```python
from build123d import *

# Parameters (mm, degrees)
RESSALTO_EXTRUS_O1_DEPTH   = 160
ESBO_O2_W                  = 7.6
ESBO_O2_H                  = 120
CORTE_EXTRUS_O1_DEPTH      = 30
CORTE_EXTRUS_O2_DEPTH      = 30
F_3DSKETCH3_R              = 2
CORTE_EXTRUS_O3_DEPTH      = 70
ESBO_O3_W                  = 45.015344868
ESBO_O3_H                  = 129.478543367
ESBO_O3_W_2                = 37.192593828
CORTE_EXTRUS_O4_DEPTH      = 41
CORTE_EXTRUS_O4_DEPTH_BACK = 22
ESBO_O4_W                  = 72.8
ESBO_O4_H                  = 73.5
CORTE_EXTRUS_O5_DEPTH      = 34
CORTE_EXTRUS_O5_DEPTH_BACK = 36


with BuildPart() as part:
    # Esboço1 → Ressalto-extrusão1 (new body)
    with BuildSketch(Plane.XY):
        with BuildLine():
            Line((-3.8, 21.821375341), (-3.8, -98.178624659))
            Line((-3.8, -98.178624659), (-5.7, -98.178624659))
            Line((-5.7, -98.178624659), (-5.360626179, -99.63308389))
            ThreePointArc((-5.360626179, -99.63308389), (-4.656141559, -100.745296045), (-3.41294376, -101.178624659))
            Line((-3.41294376, -101.178624659), (3.41294376, -101.178624659))
            ThreePointArc((3.41294376, -101.178624659), (4.656141559, -100.745296045), (5.360626179, -99.63308389))
            Line((5.360626179, -99.63308389), (5.7, -98.178624659))
            Line((5.7, -98.178624659), (3.8, -98.178624659))
            Line((3.8, -98.178624659), (3.8, 21.821375341))
            Line((3.8, 21.821375341), (5.7, 21.821375341))
            Line((5.7, 21.821375341), (4.013268169, 24.033911877))
            ThreePointArc((4.013268169, 24.033911877), (3.310139149, 24.613730366), (2.422747768, 24.821375341))
            Line((2.422747768, 24.821375341), (-2.297792791, 24.821375341))
            ThreePointArc((-2.297792791, 24.821375341), (-3.27177376, 24.568189891), (-3.999156919, 23.872736414))
            Line((-3.999156919, 23.872736414), (-5.266799243, 21.821375341))
            Line((-5.266799243, 21.821375341), (-3.8, 21.821375341))
        make_face()
    extrude(amount=RESSALTO_EXTRUS_O1_DEPTH)

    # Esboço2 → Corte-extrusão1 (cut)
    with BuildSketch(Plane.XY):
        with Locations((0, -38.178624659)):
            Rectangle(ESBO_O2_W, ESBO_O2_H)
    extrude(amount=CORTE_EXTRUS_O1_DEPTH, mode=Mode.SUBTRACT)

    # 3DSketch2 → Corte-extrusão2 (cut)
    with BuildSketch(Plane(origin=(-3.8, 21.821375341, 160), x_dir=(0.0632066956560733, -0.9980004577274705, 0), z_dir=(0, 0, -1))):
        Polygon((0, 0), (0.480370887, -7.584803479), (120.240425814, 0), (119.760054927, 7.584803479), align=None)
    extrude(amount=CORTE_EXTRUS_O2_DEPTH, mode=Mode.SUBTRACT)

    # 3DSketch3 → Corte-extrusão3 (cut)
    with BuildSketch(Plane(origin=(3.8, -38.178624659, 80), x_dir=(0, 0.7676852805184269, 0.6408270516101394), z_dir=(1, 0, 0))):
        with Locations(Location((0, 0, 0), (0, 0, 140.146481665))):
            Circle(F_3DSKETCH3_R)
        with Locations(Location((23.030558416, -19.224811548, 0), (0, 0, 140.146481665))):
            Circle(F_3DSKETCH3_R)
        with Locations(Location((-23.030558416, 19.224811548, 0), (0, 0, 140.146481665))):
            Circle(F_3DSKETCH3_R)
        with Locations(Location((-39.051234706, 0.032679535, 0), (0, 0, 140.146481665))):
            Circle(F_3DSKETCH3_R)
        with Locations(Location((-16.02067629, -19.192132013, 0), (0, 0, 140.146481665))):
            Circle(F_3DSKETCH3_R)
        with Locations(Location((7.009882125, -38.416943561, 0), (0, 0, 140.146481665))):
            Circle(F_3DSKETCH3_R)
        with Locations(Location((-6.982602808, 38.449623097, 0), (0, 0, 140.146481665))):
            Circle(F_3DSKETCH3_R)
        with Locations(Location((16.047955607, 19.224811548, 0), (0, 0, 140.146481665))):
            Circle(F_3DSKETCH3_R)
        with Locations(Location((39.078514023, 0, 0), (0, 0, 140.146481665))):
            Circle(F_3DSKETCH3_R)
    extrude(amount=-CORTE_EXTRUS_O3_DEPTH, mode=Mode.SUBTRACT)

    # Esboço3 → Corte-extrusão4 (cut, two sides)
    with BuildSketch(Plane(origin=(0, 0, 0), x_dir=(0, 0, -1), z_dir=(1, 0, 0))) as corte_extrus_o4_sk:
        with Locations((-7.492327566, -39.917896343)):
            Rectangle(ESBO_O3_W, ESBO_O3_H)
        with Locations((-148.596296914, -39.917896343)):
            Rectangle(ESBO_O3_W_2, ESBO_O3_H)
    extrude(amount=CORTE_EXTRUS_O4_DEPTH, mode=Mode.SUBTRACT)
    extrude(corte_extrus_o4_sk.sketch, amount=-CORTE_EXTRUS_O4_DEPTH_BACK, mode=Mode.SUBTRACT)

    # Esboço4 → Corte-extrusão5 (cut, two sides)
    with BuildSketch(Plane(origin=(0, 0, 0), x_dir=(0, 0, -1), z_dir=(1, 0, 0))) as corte_extrus_o5_sk:
        with Locations((-81.6, -19.928624659)):
            Rectangle(ESBO_O4_W, ESBO_O4_H)
        Polygon((-93.057510279, -86.178624659), (-62.607510279, -86.178624659), (-62.607510279, -83.253419483), (-63.607510279, -78.466022071), (-63.607510279, -73.678624659), (-92.057510279, -73.678624659), (-92.057510279, -78.466022071), (-93.057510279, -83.253419483), align=None)
    extrude(amount=CORTE_EXTRUS_O5_DEPTH, mode=Mode.SUBTRACT)
    extrude(corte_extrus_o5_sk.sketch, amount=-CORTE_EXTRUS_O5_DEPTH_BACK, mode=Mode.SUBTRACT)


solid = part.part
```
Verification items for the finished model (mm, model axes). A direction names the side the tool comes from. Round coordinates to 2 decimals unless told otherwise and drop trailing zeros. Order: outer loops, then holes, each group sorted by start corner. A loop starts at its lowest first (then second) coordinate and runs counter-clockwise, first axis right, second up. Notation, with made-up numbers: (49, 73) - (91, 73) arc R7 ccw to (91, 78) - close; hole circle Ø6 at (-8.75, -30). An arc over 180 degrees is marked (long way). Use CSV: the item, a comma, the result in double quotes.
(1) Section check C-C on z = 113.5. Record the boundary of the cut face in (x, y).
Entries:
outline,"(-5.7, -98.18) - (-5.36, -99.63) arc R2 ccw to (-3.41, -101.18) - (3.41, -101.18) arc R2 ccw to (5.36, -99.63) - (5.7, -98.18) - (3.8, -98.18) - (3.8, -56.68) - (-3.8, -56.68) - (-3.8, -98.18) - close; (-5.27, 21.82) - (-3.8, 21.82) - (-3.8, 16.82) - (3.8, 16.82) - (3.8, 21.82) - (5.7, 21.82) - (4.01, 24.03) arc R2 ccw to (2.42, 24.82) - (-2.3, 24.82) arc R2 ccw to (-4, 23.87) - close"
(2) Gauge pin test, flat ends, axial feed: pin 1 Ø5 at (y, z) = (-68.18, 80) entering from +X; pin 2 Ø6.5 at (y, z) = (-68.18, 105.04) entering from -X; pin 3 Ø1.2 at (x, z) = (-4.5, 73.5) entering from -Y; pin 4 Ø8 at (y, z) = (10.5, 83.5) entering from -X. Record the tip position at first contact, or that the pin passes through.
Entries:
pin 1,"x = 3.8"
pin 2,"x = -3.8"
pin 3,"y = -101.12"
pin 4,"through"
(3) Thickness scan on probe 1 along Y at (x, z) = (0.75, 84); probe 2 along Y at (x, z) = (1.25, 61); probe 3 along Z at (x, y) = (-1, 11.5). Record the ranges inside material, lowest first. Write a range as from..to.
Entries:
probe 1,"-101.18..-86.18, -73.68..-56.68, 16.82..24.82"
probe 2,"-101.18..-56.68, 16.82..24.82"
probe 3,"30..45.2, 118..130"
(4) Section check A-A on z = 70. Record the boundary of the cut face in (x, y), and give its area (3 significant figures).
Entries:
outline,"(-5.7, -98.18) - (-5.36, -99.63) arc R2 ccw to (-3.41, -101.18) - (3.41, -101.18) arc R2 ccw to (5.36, -99.63) - (5.7, -98.18) - (3.8, -98.18) - (3.8, -86.18) - (-3.8, -86.18) - (-3.8, -98.18) - close; (-5.27, 21.82) - (-3.8, 21.82) - (-3.8, 16.82) - (3.8, 16.82) - (3.8, 21.82) - (5.7, 21.82) - (4.01, 24.03) arc R2 ccw to (2.42, 24.82) - (-2.3, 24.82) arc R2 ccw to (-4, 23.87) - close; (-3.8, -73.68) - (3.8, -73.68) - (3.8, -56.68) - (-3.8, -56.68) - close"
area,"316 mm^2"
(5) Section check D-D on z = 80. Record the boundary of the cut face in (x, y).
Entries:
outline,"(-5.7, -98.18) - (-5.36, -99.63) arc R2 ccw to (-3.41, -101.18) - (3.41, -101.18) arc R2 ccw to (5.36, -99.63) - (5.7, -98.18) - (3.8, -98.18) - (3.8, -86.18) - (-3.8, -86.18) - (-3.8, -98.18) - close; (-5.27, 21.82) - (-3.8, 21.82) - (-3.8, 16.82) - (3.8, 16.82) - (3.8, 21.82) - (5.7, 21.82) - (4.01, 24.03) arc R2 ccw to (2.42, 24.82) - (-2.3, 24.82) arc R2 ccw to (-4, 23.87) - close; (-3.8, -73.68) - (3.8, -73.68) - (3.8, -70.18) - (-3.8, -70.18) - close; (-3.8, -66.18) - (3.8, -66.18) - (3.8, -56.68) - (-3.8, -56.68) - close"
(6) Section check B-B on y = -29. Record the boundary of the cut face in (x, z).
Entries:
outline,"(-3.8, 30) - (3.8, 30) - (3.8, 45.2) - (-3.8, 45.2) - close; (-3.8, 118) - (3.8, 118) - (3.8, 130) - (-3.8, 130) - close"
(7) Mould release check, pull along Y, two halves, no side actions. Record for faces 1 (the face through (-1, -39, 130)), 2 (the face through (0, 16.821, 82)), 3 (the face through (0, 24.821, 79)): released by +Y, released by -Y, zero draft, split by the parting line, or undercut.
Entries:
face 1,"zero draft"
face 2,"undercut"
face 3,"released by +Y"
(8) Access from +Z, -Z, +X, -X, +Y, -Y to the whole of each face (thin tool, end or side, straight path). Record for faces 4 (the face through (-1, -39, 30)), 5 (the face through (-3.8, -64, 79)), 6 (the face through (0, -85, 62.608)), 7 (the face through (3.8, -66, 79)).
Entries:
face 4,"-Z, +X, -X, +Y, -Y"
face 5,"+Z, -Z, -X"
face 6,"+X, -X"
face 7,"+Z, -Z, +X"
